Verification items for the finished model (mm, model axes). A direction names the side the tool comes from. Round coordinates to 2 decimals unless told otherwise and drop trailing zeros. Write each loop counter-clockwise with the first axis right and the second up, starting at its lowest first coordinate (ties: lowest second). Pieces come first, ordered by that corner, then holes. Notation, with made-up numbers: M 0.25,39.25 L 40.25,39.25 A15 ccw 40.25,54.25 Z; hole C 39.25,58 d7. An arc over 180 degrees is marked long. One line per item, written item: value. Start each with the question number.
Item 1: Gauge pin test, flat ends, axial feed: pin 1 (3.5 mm diameter, centred on x = -42.87, z = 24.75, fed in from -Y) (1 decimal); pin 2 (2 mm diameter, centred on y = 9.5, z = -22.5, fed in from -X); pin 3 (2 mm diameter, centred on y = 11, z = 35, fed in from +X). Record the tip position at first contact, or that the pin passes through.
Item 2: Section check C-C, the plane z = -18. Record the cut outline in (x, y).
Item 3: Tool access check on faces 4 (the face through (-55.645, 8.944, -12.356)), 5 (the face through (-27.27, 13, 50.23)). Record the directions out of +Z, -Z, +X, -X, +Y, -Y that give a thin tool (end or side, any length) a straight path to the whole face; none if there is none.
Item 4: Thickness scan on probe 1 along X at (y, z) = (10.25, 0); probe 2 along Y at (x, z) = (-19, 14); probe 3 along X at (y, z) = (12.75, 23). Record the ranges inside material, lowest first. Write a range as from..to.
Item 5: Section check D-D, the plane y = 10.25. Record the cut outline in (x, z), then the cut area to 3 significant figures.
Item 6: Section check A-A, the plane z = 0. Record the cut outline in (x, y).
Item 7: Draft check along Y on faces 1 (the face through (-12, 5, -1)), 2 (the face through (-28.65, 6.95, 52.12)), 3 (the face through (0.088, 2.535, -51.498)). Enter one of: +Y half, -Y half, draft (parallel to the pull), parting line (faces both ways), or undercut.
Item 8: Section check B-B, the plane x = 0. Record the cut outline in (y, z).
from build123d import *

# Parameters (mm, degrees)
SKETCH1_R               = 62
BOSS_EXTRUDE1_DEPTH     = 5
SKETCH2_R               = 2
CUT_EXTRUDE1_DEPTH      = 5
CIRPATTERN1_COUNT       = 2
CIRPATTERN1_ANGLE       = 120
MIRROR1_COPY_1_SKETCH_R = 2
MIRROR1_COPY_1_DEPTH    = 5
SKETCH5_R               = 62
SKETCH5_R_2             = 57
BOSS_EXTRUDE2_DEPTH     = 8
CUT_EXTRUDE2_START      = -90
SKETCH6_R               = 1.25
CUT_EXTRUDE2_DEPTH      = 192
CIRPATTERN2_COUNT       = 2
CIRPATTERN2_ANGLE       = 90
SKETCH7_R               = 3
CUT_EXTRUDE3_DEPTH      = 10


with BuildPart() as part:
    # Sketch1 → Boss-Extrude1 (new body)
    with BuildSketch(Plane(origin=(0, 0, 0), x_dir=(1, 0, 0), z_dir=(0, 1, 0))):
        with Locations(Location((0, 0, 0), (0, 0, 270))):
            Circle(SKETCH1_R)
    extrude(amount=BOSS_EXTRUDE1_DEPTH)

    # Sketch2 → Cut-Extrude1 (cut)
    with BuildSketch(Plane(origin=(0, 5, 0), x_dir=(1, 0, 0), z_dir=(0, 1, 0))):
        with Locations(Location((0, 49.5, 0), (0, 0, 270))):
            Circle(SKETCH2_R)
    cut_extrude1 = extrude(amount=-CUT_EXTRUDE1_DEPTH, mode=Mode.SUBTRACT)

    # CirPattern1: Cut-Extrude1 ×2 about axis
    cirpattern1_axis = Axis((0, 5, 0), (0, 1, 0))
    for i in range(1, CIRPATTERN1_COUNT):
        add(cut_extrude1.rotate(cirpattern1_axis, i * CIRPATTERN1_ANGLE / (CIRPATTERN1_COUNT - 1)), mode=Mode.SUBTRACT)

    # Mirror1: Cut-Extrude1 across plane
    add(cut_extrude1.mirror(Plane(origin=(0, 0, 0), x_dir=(-0.49999999999999806, 0, 0.8660254037844398), z_dir=(-0.8660254037844398, 0, -0.49999999999999806))), mode=Mode.SUBTRACT)

    # Mirror1 copy 1 sketch → Mirror1 copy 1 (cut)
    with BuildSketch(Plane(origin=(0, 5, 0), x_dir=(1, 0, 0), z_dir=(0, 1, 0))):
        with Locations((0, -49.5)):
            Circle(MIRROR1_COPY_1_SKETCH_R)
    extrude(amount=-MIRROR1_COPY_1_DEPTH, mode=Mode.SUBTRACT)

    # Sketch5 → Boss-Extrude2 (add)
    with BuildSketch(Plane(origin=(0, 5, 0), x_dir=(1, 0, 0), z_dir=(0, 1, 0))):
        with Locations(Location((0, 0, 0), (0, 0, 270))):
            Circle(SKETCH5_R)
        with Locations(Location((0, 0, 0), (0, 0, 270))):
            Circle(SKETCH5_R_2, mode=Mode.SUBTRACT)
    extrude(amount=BOSS_EXTRUDE2_DEPTH)

    # Sketch6 → Cut-Extrude2 (cut)
    with BuildSketch(Plane(origin=(0, 0, 0), x_dir=(-0.49999999999999806, 0, 0.8660254037844398), z_dir=(-0.8660254037844398, 0, -0.49999999999999806)).offset(CUT_EXTRUDE2_START)):
        with Locations(Location((0, 7, 0), (0, 0, 180))):
            Circle(SKETCH6_R)
    cut_extrude2 = extrude(amount=CUT_EXTRUDE2_DEPTH, mode=Mode.SUBTRACT)

    # CirPattern2: Cut-Extrude2 ×2 about axis
    cirpattern2_axis = Axis((0, 13, 0), (0, 1, 0))
    for i in range(1, CIRPATTERN2_COUNT):
        add(cut_extrude2.rotate(cirpattern2_axis, i * CIRPATTERN2_ANGLE / (CIRPATTERN2_COUNT - 1)), mode=Mode.SUBTRACT)

    # Sketch7 → Cut-Extrude3 (cut)
    with BuildSketch(Plane(origin=(0, 5, 0), x_dir=(1, 0, 0), z_dir=(0, 1, 0))):
        with Locations(Location((0, 0, 0), (0, 0, 270))):
            Circle(SKETCH7_R)
    extrude(amount=-CUT_EXTRUDE3_DEPTH, mode=Mode.SUBTRACT)


solid = part.part
Response values:
1. pin 1: passes through
1. pin 2: stops at x = -58.15
1. pin 3: stops at x = 51.85
2. outline: M -59.33,0 L 59.33,0 L 59.33,13 L 54.08,13 L 54.08,5 L -54.08,5 L -54.08,13 L -59.33,13 Z
3. face 4: +Y
3. face 5: +Z, -Z, +X, -X, +Y
4. probe 1: x = -62..-57, 57..62
4. probe 2: y = 0..5
4. probe 3: x = -57.58..-52.15, 52.15..57.58
5. outline: C 0,0 d124; hole C 0,0 d114
5. area: 1,870 mm2
6. outline: M -62,0 L -3,0 L -3,5 L -57,5 L -57,13 L -62,13 Z; M 3,0 L 62,0 L 62,13 L 57,13 L 57,5 L 3,5 Z
7. face 1: +Y half
7. face 2: undercut
7. face 3: draft
8. outline: M 0,-62 L 13,-62 L 13,-57 L 5,-57 L 5,-51.5 L 0,-51.5 Z; M 0,-47.5 L 5,-47.5 L 5,-3 L 0,-3 Z; M 0,3 L 5,3 L 5,47.5 L 0,47.5 Z; M 0,51.5 L 5,51.5 L 5,57 L 13,57 L 13,62 L 0,62 Z
